Geometry: see drawing. Coordinates: mm, zero at the bounding-box minimum. A direction names the side the tool comes from. Coordinates: 2 decimals unless noted, no trailing zeros. Loops run counter-clockwise (first coordinate to the right, second up) from the corner with the lowest first, then second, coordinate; pieces in that order, holes last. Notation, with made-up numbers: (76.25, -37) -> (106.25, -37) arc R35 cw to (106.25, 0) -> close; hole circle Ø2 at (9.5, 70.5). An arc over 180 degrees is marked (long way). One line per question, with ' | ' between items. Start each with the question number.
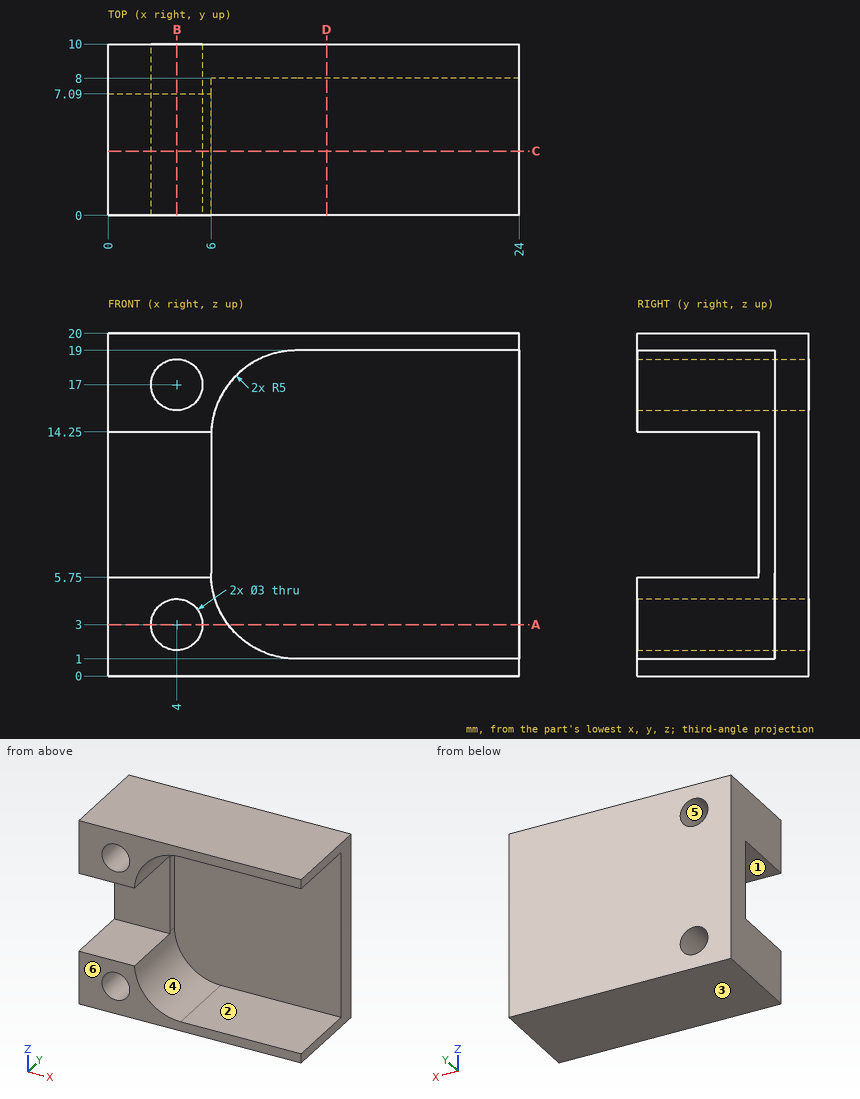
(1) Cut plane D-D, the plane x = 12.75. Return the cut outline in (y, z).
(2) Cut plane C-C, the plane y = 3.75. Return the cut outline in (x, z).
(3) Cut plane A-A, the plane z = 3. Return the cut outline in (x, y).
(4) Contact query for flat-ended pins moving along their axis: pin 1 Ø0.7 at (y, z) = (7.5, 9.5) entering from +X; pin 2 Ø4 at (x, z) = (10.5, 11) entering from -Y. Output: stop coordinate, or through.
(5) Cut plane B-B, the plane x = 4. Return the cut outline in (y, z).
(6) Draft query along X for the marked faces 4, 5 and 6. Return one class per face: pulls with the +X half, pulls with the -X half, needs draft (parallel to the pull), parting line crosses it, or undercut.
(7) Ray query, L1, parallel to Z at x = 4, y = 6.75; L2, parallel to Z at x = 18.25, y = 4.5; L3, parallel to Y at x = 6.75, z = 8. Return the intervals inside material, ascending.
(8) Access query for the marked faces 1, 2 and 3. Directions: +Z, -Z, +X, -X, +Y, -Y. A direction counts if a zero-diameter tool reaches every point of the face in a straight line with its end or side. Return the directions, or none.
Here are the results:
1) outline: (0, 0) -> (10, 0) -> (10, 20) -> (0, 20) -> (0, 19) -> (8, 19) -> (8, 1) -> (0, 1) -> close
2) outline: (0, 0) -> (24, 0) -> (24, 1) -> (11, 1) arc R5 cw to (6.01, 5.75) -> (0, 5.75) -> close; (0, 14.25) -> (6.01, 14.25) arc R5 cw to (11, 19) -> (24, 19) -> (24, 20) -> (0, 20) -> close; hole circle Ø3 at (4, 3); hole circle Ø3 at (4, 17)
3) outline: (0, 0) -> (2.5, 0) -> (2.5, 10) -> (0, 10) -> close; (5.5, 0) -> (7, 0) -> (7, 8) -> (24, 8) -> (24, 10) -> (5.5, 10) -> close
4) pin 1: stops at x = 6 | pin 2: stops at y = 8
5) outline: (0, 0) -> (10, 0) -> (10, 1.5) -> (0, 1.5) -> close; (0, 4.5) -> (10, 4.5) -> (10, 15.5) -> (0, 15.5) -> (0, 14.25) -> (7.09, 14.25) -> (7.09, 5.75) -> (0, 5.75) -> close; (0, 18.5) -> (10, 18.5) -> (10, 20) -> (0, 20) -> close
6) face 4: pulls with the +X half | face 5: undercut | face 6: needs draft
7) L1: z = 0 to 1.5, 4.5 to 5.75, 14.25 to 15.5, 18.5 to 20 | L2: z = 0 to 1, 19 to 20 | L3: y = 8 to 10
8) face 1: +X, -X, -Y | face 2: +X, -Y | face 3: -Z, +X, -X, +Y, -Y
